Read the model definition and answer for the solid it produces. Units are mm, in the model's axes. A direction names the side the tool comes from. Coordinates: 2 decimals unless noted, no trailing zeros. Order: outer loops, then holes, each group sorted by start corner. A loop starts at its lowest first (then second) coordinate and runs counter-clockwise, first axis right, second up. Notation, with made-up numbers: M 6.5,81 L 58.5,81 A8 cw 58.5,88 Z; hole C 15,-37 d9. An arc over 180 degrees is marked long. Use a Markdown table: item, result. Add a question column.
1) Find section B-B on x = 5.75. Write down the section's boundary in (y, z), plus the area to 3 significant figures.
2) Find the intervals of material crossed by probe 1 along Y at (x, z) = (1.75, 2.5); probe 2 along Z at (x, y) = (5.25, 2.25), in increasing order. Write a range as [from, to].
3) The mould has two halves that part along Y. Classify faces 3 (the face through (9.57, 9.55, 5.42)), 4 (the face through (0, -10, 5)), 5 (the face through (9, 0, 6)): released by +Y, released by -Y, zero draft, split by the parting line, or undercut.
4) For faces 1 (the face through (9.55, -9.57, 5.58)), 2 (the face through (-9, 0, 6)), determine the directions among +Z, -Z, +X, -X, +Y, -Y from which every point of the face is accessible in a straight line to the end or side of a thin tool.
5) This flat-tipped pin is pushed along its axis until it touches: pin 1 Ø1 at (x, y) = (-5, 2.5) entering from +Z. Where does it stop, or does it pass through?
6) Find section A-A on z = 3. Write down the section's boundary in (x, y).
7) Find section C-C on y = 8.75. Write down the section's boundary in (x, z), plus the area to 3 significant figures.
from build123d import *

# Parameters (mm, degrees)
F0_W     = 20
F0_H     = 20
F1_DEPTH = 1
F2_W     = 20
F2_H     = 20
F2_W_2   = 18
F2_H_2   = 18
F3_DEPTH = 10
F4_R     = 1.5
F5_R     = 0.5
F6_R     = 1.5
F7_R     = 1.5
F8_R     = 1.5
F9_R     = 0.5
F10_R    = 0.5
F11_R    = 0.5


with BuildPart() as f1:
    # F0 (on Top) → F1 (new body)
    with BuildSketch(Plane.XY):
        Rectangle(F0_W, F0_H)
    extrude(amount=F1_DEPTH)

    # F2 (on face) → F3 (join)
    with BuildSketch(Plane.XY.offset(1)):
        Rectangle(F2_W, F2_H)
        Rectangle(F2_W_2, F2_H_2, mode=Mode.SUBTRACT)
    extrude(amount=F3_DEPTH)

    # F4
    f4_edges = [f1.edges().sort_by_distance(p)[0] for p in [
        (10, -10, 5.5),
    ]]
    fillet(f4_edges, radius=F4_R)

    # F5
    f5_edges = [f1.edges().sort_by_distance(p)[0] for p in [
        (9, -9, 6),
    ]]
    fillet(f5_edges, radius=F5_R)

    # F6
    f6_edges = [f1.edges().sort_by_distance(p)[0] for p in [
        (10, 10, 5.5),
    ]]
    fillet(f6_edges, radius=F6_R)

    # F7
    f7_edges = [f1.edges().sort_by_distance(p)[0] for p in [
        (-10, 10, 5.5),
    ]]
    fillet(f7_edges, radius=F7_R)

    # F8
    f8_edges = [f1.edges().sort_by_distance(p)[0] for p in [
        (-10, -10, 5.5),
    ]]
    fillet(f8_edges, radius=F8_R)

    # F9
    f9_edges = [f1.edges().sort_by_distance(p)[0] for p in [
        (-9, 9, 6),
    ]]
    fillet(f9_edges, radius=F9_R)

    # F10
    f10_edges = [f1.edges().sort_by_distance(p)[0] for p in [
        (9, 9, 6),
    ]]
    fillet(f10_edges, radius=F10_R)

    # F11
    f11_edges = [f1.edges().sort_by_distance(p)[0] for p in [
        (-9, -9, 6),
    ]]
    fillet(f11_edges, radius=F11_R)


solid = f1.part
Check result:
| question | item | result |
|---|---|---|
| 1 | outline | M -10,0 L 10,0 L 10,11 L 9,11 L 9,1 L -9,1 L -9,11 L -10,11 Z |
| 1 | area | 40.0 mm2 |
| 2 | probe 1 | y = [-10, -9], [9, 10] |
| 2 | probe 2 | z = [0, 1] |
| 3 | face 3 | released by +Y |
| 3 | face 4 | released by -Y |
| 3 | face 5 | undercut |
| 4 | face 1 | +Z, -Z, +X, -Y |
| 4 | face 2 | +Z |
| 5 | pin 1 | stops at z = 1 |
| 6 | outline | M -10,-8.5 A1.5 ccw -8.5,-10 L 8.5,-10 A1.5 ccw 10,-8.5 L 10,8.5 A1.5 ccw 8.5,10 L -8.5,10 A1.5 ccw -10,8.5 Z; hole M -9,-8.5 A0.5 ccw -8.5,-9 L 8.5,-9 A0.5 ccw 9,-8.5 L 9,8.5 A0.5 ccw 8.5,9 L -8.5,9 A0.5 ccw -9,8.5 Z |
| 7 | outline | M -9.98,0 L 9.98,0 L 9.98,11 L 8.93,11 L 8.93,1 L -8.93,1 L -8.93,11 L -9.98,11 Z |
| 7 | area | 40.9 mm2 |
